Verification items for the finished model (mm, model axes). Give positions to 0.01 mm unless a question says otherwise; leave off trailing zeros. Order: outer loops, then holes, each group sorted by start corner. A loop starts at its lowest first (then second) coordinate and runs counter-clockwise, first axis right, second up. Notation, with made-up numbers: (49, 54.25) - (59, 54.25) arc R30 ccw to (59, 79.25) - close; hole circle Ø5 at (64, 38.25). An arc over 180 degrees is marked (long way). Answer as a JSON object with one key per item and string values. Group by question number.
(1) Depth check by flat-ended pin: pin 1 Ø0.8 at (x, y) = (41.5, -0.5) entering from +Z; pin 2 Ø0.8 at (y, z) = (-0.5, -37) entering from -X; pin 3 Ø0.8 at (x, y) = (-41.5, -0.5) entering from -Z. Enter the tip coordinate at first touch or a pass-through.
(2) Section check A-A (z = -125). Record the boundary of the cut face in (x, y), then the cut area to 3 significant figures.
(3) Thickness scan on line 1 (Z direction, x = 0, y = 8); line 2 (X direction, y = 21.5, z = -125); line 3 (Y direction, x = -75.5, z = -101.5). Record the ranges inside material, lowest first.
(4) Section check C-C (z = -75.5). Record the boundary of the cut face in (x, y), then the cut area to 3 significant figures.
(5) Section check B-B (x = -75). Record the boundary of the cut face in (y, z), then the cut area to 3 significant figures.
```python
from build123d import *

# Parameters (mm, degrees)
ESBO_O1_W                    = 200
ESBO_O1_H                    = 250
RESSALTO_EXTRUS_O1_DEPTH     = 50
FURO_DE_DI_METRO_16_0_16_1_D = 16
PADR_O_LINEAR1_COUNT         = 3
PADR_O_LINEAR1_PITCH         = 30
PADR_O_LINEAR1_COUNT_DIR2    = 2
PADR_O_LINEAR1_PITCH_DIR2    = 120
ESBO_O7_W                    = 1.03
ESBO_O7_H                    = 10.3
RESSALTO_EXTRUS_O2_DEPTH     = 1


with BuildPart() as part:
    # Esboço1 → Ressalto-extrusão1 (new body)
    with BuildSketch(Plane(origin=(0, 0, 0), x_dir=(1, 0, 0), z_dir=(0, 1, 0))):
        with Locations((0, 125)):
            Rectangle(ESBO_O1_W, ESBO_O1_H)
    extrude(amount=RESSALTO_EXTRUS_O1_DEPTH)

    # Furo de diâmetro Ø16.0 (16)1 (through all)
    with Locations(Plane(origin=(0, 50, 0), x_dir=(1, 0, 0), z_dir=(0, 1, 0))):
        with Locations((0, 125)):
            Hole(FURO_DE_DI_METRO_16_0_16_1_D / 2)

    # Esboço5 → Corte-Revolução1 (revolve, cut)
    with BuildSketch(Plane.XZ):
        with BuildLine():
            Line((0, -27), (0, -223))
            ThreePointArc((0, -223), (2.121320344, -222.121320344), (3, -220))
            Line((3, -220), (3, -30))
            ThreePointArc((3, -30), (2.121320344, -27.878679656), (0, -27))
        make_face()
    revolve(axis=Axis((0, 0, -27), (0, 0, -1)), mode=Mode.SUBTRACT)

    # Esboço6 → Corte-Revolução2 (revolve, cut)
    with BuildSketch(Plane.XZ):
        with BuildLine():
            Line((-9, -34.85), (0, -34.85))
            Line((0, -34.85), (0, -31.85))
            Line((0, -31.85), (-6, -31.85))
            ThreePointArc((-6, -31.85), (-8.121320344, -32.728679656), (-9, -34.85))
        make_face()
    corte_revolu_o2 = revolve(axis=Axis((-9, 0, -34.85), (1, 0, 0)), mode=Mode.SUBTRACT)

    # Padrão linear1: Corte-Revolu_o2 3 × 2
    with Locations(*[Vector(0, 0, -1) * (i * PADR_O_LINEAR1_PITCH) + Vector(0, 0, -1) * (j * PADR_O_LINEAR1_PITCH_DIR2) for i in range(PADR_O_LINEAR1_COUNT) for j in range(PADR_O_LINEAR1_COUNT_DIR2) if (i, j) != (0, 0)]):
        add(corte_revolu_o2, mode=Mode.SUBTRACT)

    # Espelhar1: Corte-Revolução2 across plane
    add(corte_revolu_o2.mirror(Plane(origin=(0, 0, 0), x_dir=(0, 0, 1), z_dir=(1, 0, 0))), mode=Mode.SUBTRACT)

    # Espelhar1 copy 1 sketch → Espelhar1 copy 1 (revolve, cut)
    with BuildSketch(Plane(origin=(0, 0, -120), x_dir=(-1, 0, 0), z_dir=(0, -1, 0))):
        with BuildLine():
            Line((-9, 34.85), (0, 34.85))
            Line((0, 34.85), (0, 31.85))
            Line((0, 31.85), (-6, 31.85))
            ThreePointArc((-6, 31.85), (-8.121320344, 32.728679656), (-9, 34.85))
        make_face()
    revolve(axis=Axis((9, 0, -154.85), (1, 0, 0)), mode=Mode.SUBTRACT)

    # Espelhar1 copy 2 sketch → Espelhar1 copy 2 (revolve, cut)
    with BuildSketch(Plane(origin=(0, 0, -30), x_dir=(-1, 0, 0), z_dir=(0, -1, 0))):
        with BuildLine():
            Line((-9, 34.85), (0, 34.85))
            Line((0, 34.85), (0, 31.85))
            Line((0, 31.85), (-6, 31.85))
            ThreePointArc((-6, 31.85), (-8.121320344, 32.728679656), (-9, 34.85))
        make_face()
    revolve(axis=Axis((9, 0, -64.85), (1, 0, 0)), mode=Mode.SUBTRACT)

    # Espelhar1 copy 3 sketch → Espelhar1 copy 3 (revolve, cut)
    with BuildSketch(Plane(origin=(0, 0, -150), x_dir=(-1, 0, 0), z_dir=(0, -1, 0))):
        with BuildLine():
            Line((-9, 34.85), (0, 34.85))
            Line((0, 34.85), (0, 31.85))
            Line((0, 31.85), (-6, 31.85))
            ThreePointArc((-6, 31.85), (-8.121320344, 32.728679656), (-9, 34.85))
        make_face()
    revolve(axis=Axis((9, 0, -184.85), (1, 0, 0)), mode=Mode.SUBTRACT)

    # Espelhar1 copy 4 sketch → Espelhar1 copy 4 (revolve, cut)
    with BuildSketch(Plane(origin=(0, 0, -60), x_dir=(-1, 0, 0), z_dir=(0, -1, 0))):
        with BuildLine():
            Line((-9, 34.85), (0, 34.85))
            Line((0, 34.85), (0, 31.85))
            Line((0, 31.85), (-6, 31.85))
            ThreePointArc((-6, 31.85), (-8.121320344, 32.728679656), (-9, 34.85))
        make_face()
    revolve(axis=Axis((9, 0, -94.85), (1, 0, 0)), mode=Mode.SUBTRACT)

    # Espelhar1 copy 5 sketch → Espelhar1 copy 5 (revolve, cut)
    with BuildSketch(Plane(origin=(0, 0, -180), x_dir=(-1, 0, 0), z_dir=(0, -1, 0))):
        with BuildLine():
            Line((-9, 34.85), (0, 34.85))
            Line((0, 34.85), (0, 31.85))
            Line((0, 31.85), (-6, 31.85))
            ThreePointArc((-6, 31.85), (-8.121320344, 32.728679656), (-9, 34.85))
        make_face()
    revolve(axis=Axis((9, 0, -214.85), (1, 0, 0)), mode=Mode.SUBTRACT)

    # Esboço7 → Ressalto-extrusão2 (add)
    with BuildSketch(Plane.XZ):
        with Locations((-41.415, -35.15)):
            Rectangle(ESBO_O7_W, ESBO_O7_H)
        with Locations((-41.415, -65.15)):
            Rectangle(ESBO_O7_W, ESBO_O7_H)
        with Locations((-41.415, -95.15)):
            Rectangle(ESBO_O7_W, ESBO_O7_H)
        with Locations((-41.415, -154.85)):
            Rectangle(ESBO_O7_W, ESBO_O7_H)
        with Locations((-41.415, -184.85)):
            Rectangle(ESBO_O7_W, ESBO_O7_H)
        with Locations((-41.415, -214.85)):
            Rectangle(ESBO_O7_W, ESBO_O7_H)
        with Locations((41.415, -214.85)):
            Rectangle(ESBO_O7_W, ESBO_O7_H)
        with Locations((41.415, -184.85)):
            Rectangle(ESBO_O7_W, ESBO_O7_H)
        with Locations((41.415, -154.85)):
            Rectangle(ESBO_O7_W, ESBO_O7_H)
        with Locations((41.415, -95.15)):
            Rectangle(ESBO_O7_W, ESBO_O7_H)
        with Locations((41.415, -65.15)):
            Rectangle(ESBO_O7_W, ESBO_O7_H)
        with Locations((41.415, -35.15)):
            Rectangle(ESBO_O7_W, ESBO_O7_H)
    extrude(amount=RESSALTO_EXTRUS_O2_DEPTH)


solid = part.part
```
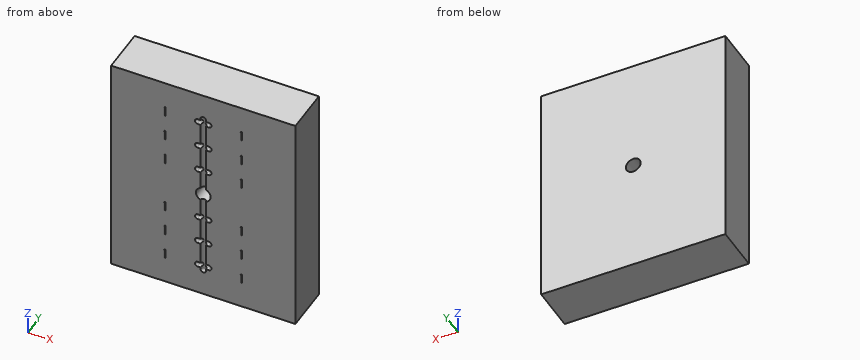
Solutions:
{
 "1": {"pin 1": "stops at z = -30", "pin 2": "stops at x = -41.93", "pin 3": "stops at z = -220"},
 "2": {"outline": "(-100, 0) - (-8, 0) - (-8, 50) - (-100, 50) - close; (8, 0) - (100, 0) - (100, 50) - (8, 50) - close", "area": "9,200 mm2"},
 "3": {"line 1": "z = -250 to -133, -117 to 0", "line 2": "x = -100 to -8, 8 to 100", "line 3": "y = 0 to 50"},
 "4": {"outline": "(-100, 0) - (-3, 0) arc R3 cw to (3, 0) - (100, 0) - (100, 50) - (-100, 50) - close", "area": "9,990 mm2"},
 "5": {"outline": "(0, -250) - (50, -250) - (50, 0) - (0, 0) - close", "area": "12,500 mm2"}
}
